Check sheet for the modelled part. Datum: model origin and axes. Units: mm. Round coordinates to 2 decimals unless told otherwise and drop trailing zeros. Order: outer loops, then holes, each group sorted by start corner. A loop starts at its lowest first (then second) coordinate and runs counter-clockwise, first axis right, second up. Notation, with made-up numbers: (27, -1) -> (59, -1) arc R15 cw to (59, 14) -> close; hole circle Ø6 at (42.25, 26). An arc over 180 degrees is marked (long way). Answer in a Markdown table with one row per item. Add a question column.
1. Depth check by flat-ended pin: P1, Ø1.5, axis at x = 3, y = 205.5, coming from the +Z side; P2, Ø8, axis at y = 165.5, z = 7.5, coming from the +X side; P3, Ø2, axis at y = 108, z = 8, coming from the -X side; P4, Ø3, axis at x = 9.5, z = 5, coming from the +Y side. Enter the tip coordinate at first touch or a pass-through.
2. Sectioned sample at C-C, the plane y = 180.5. Record the boundary of the cut face in (x, z), then the cut area to 3 significant figures.
3. Sectioned sample at B-B, the plane x = 0. Record the boundary of the cut face in (y, z).
4. Sectioned sample at A-A, the plane z = 0. Record the boundary of the cut face in (x, y).
5. Draft check along Z on faces 1 (the cylindrical face through (-10.648, 128.856, -13.887)), 2 (the flat face through (14, 261.349, 2)), 3 (the cylindrical face through (-13.47, 128.85, -2.99)). Enter one of: +Z half, -Z half, draft (parallel to the pull), parting line (faces both ways), or undercut.
6. Material ranges on L1, parallel to X at y = 59, z = -11.5; L2, parallel to X at y = 72, z = 0; L3, parallel to Z at x = -6.5, y = 212.5, recorded low to high. Write a range as from..to.
```python
from build123d import *

# Parameters (mm, degrees)
SKETCH1_R           = 17.5
BOSS_EXTRUDE1_DEPTH = 261.349292
SKETCH2_R           = 13.796851261
CUT_EXTRUDE1_DEPTH  = 263.518480166
CHAMFER1_SIZE       = 0.785714


with BuildPart() as part:
    # Sketch1 → Boss-Extrude1 (new body)
    with BuildSketch(Plane(origin=(0, 0, 0), x_dir=(1, 0, 0), z_dir=(0, 1, 0))):
        with Locations(Location((0, 0, 0), (0, 0, 270))):
            Circle(SKETCH1_R)
    extrude(amount=BOSS_EXTRUDE1_DEPTH)

    # Sketch2 → Cut-Extrude1 (cut, through all)
    with BuildSketch(Plane(origin=(0, 0, 0), x_dir=(1, 0, 0), z_dir=(0, 1, 0))):
        with Locations(Location((0, 0, 0), (0, 0, 270))):
            Circle(SKETCH2_R)
    extrude(amount=CUT_EXTRUDE1_DEPTH, mode=Mode.SUBTRACT)

    # Chamfer1
    chamfer1_edges = [part.edges().sort_by_distance(p)[0] for p in [
        (0, 0, -17.5),
        (0, 261.349292, -17.5),
    ]]
    chamfer(chamfer1_edges, length=CHAMFER1_SIZE)


solid = part.part
```
Answer key:
| question | item | result |
|---|---|---|
| 1 | P1 | stops at z = 17.35 |
| 1 | P2 | stops at x = 17.15 |
| 1 | P3 | stops at x = -16.04 |
| 1 | P4 | passes through |
| 2 | outline | circle Ø35 at (0, 0); hole circle Ø27.59 at (0, 0) |
| 2 | area | 364 mm² |
| 3 | outline | (0, -16.71) -> (0.79, -17.5) -> (260.56, -17.5) -> (261.35, -16.71) -> (261.35, -13.8) -> (0, -13.8) -> close; (0, 13.8) -> (261.35, 13.8) -> (261.35, 16.71) -> (260.56, 17.5) -> (0.79, 17.5) -> (0, 16.71) -> close |
| 4 | outline | (-17.5, 0.79) -> (-16.71, 0) -> (-13.8, 0) -> (-13.8, 261.35) -> (-16.71, 261.35) -> (-17.5, 260.56) -> close; (13.8, 0) -> (16.71, 0) -> (17.5, 0.79) -> (17.5, 260.56) -> (16.71, 261.35) -> (13.8, 261.35) -> close |
| 5 | face 1 | parting line |
| 5 | face 2 | draft |
| 5 | face 3 | undercut |
| 6 | L1 | x = -13.19..-7.62, 7.62..13.19 |
| 6 | L2 | x = -17.5..-13.8, 13.8..17.5 |
| 6 | L3 | z = -16.25..-12.17, 12.17..16.25 |
